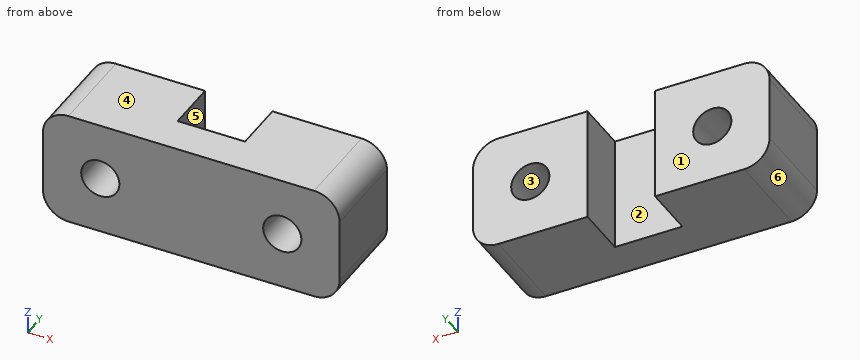
Autodesk Inventor part; units mm, degrees
ref_plane "YZ Plane" through (0, 0, 0) normal (1, 0, 0) x (0, 1, 0)
ref_plane "XZ Plane" through (0, 0, 0) normal (0, 1, 0) x (-1, 0, 0)
ref_plane "XY Plane" through (0, 0, 0) normal (0, 0, 1) x (1, 0, 0)
sketch "Sketch1" plane through (0, 0, 0) normal (0, 0, 1) x (1, 0, 0)
  line L0 (-4.3298, 0.4357) -> (0.9702, 0.4357)
  line L1 (0.9702, 0.4357) -> (0.9702, 4.5357)
  line L2 (-4.3298, 0.4357) -> (-4.3298, 4.5357)
  line L3 (-4.3298, 4.5357) -> (-13.3298, 4.5357)
  line L4 (0.9702, 4.5357) -> (9.9702, 4.5357)
  line L5 (-13.3298, 4.5357) -> (-13.3298, -2.5643)
  line L6 (-13.3298, -2.5643) -> (9.9702, -2.5643)
  line L7 (9.9702, -2.5643) -> (9.9702, 4.5357)
  point P0 (0, 0)
  dimension "d0" = 5.3
  dimension "d1" = 4.1
  dimension "d2" = 9
  dimension "d3" = 9
  dimension "d4" = 3
  dimension "d5" = 4.1
extrude "Extrusion1" add sketch "Sketch1" along normal blind 9
sketch "Sketch2" plane through (-13.3298, 4.5357, 0) normal (0, 1, 0) x (1, 0, 0)
  line L0 (0, 0) -> (9, 0)
  line L1 (0, 0) -> (0, -9)
  line L2 (9, -9) -> (0, -9)
  line L3 (9, 0) -> (9, -9)
  line L4 (14.3, 0) -> (23.3, 0)
  line L5 (14.3, 0) -> (14.3, -9)
  line L6 (23.3, -9) -> (14.3, -9)
  line L7 (23.3, 0) -> (23.3, -9)
  point P0 (13.3298, 0)
  point P1 (4.5, -4.5)
  point P2 (18.8, -4.5)
  dimension "d8" = 9
  dimension "d9" = 9
  dimension "d10" = 4.5
  dimension "d11" = 4.5
  dimension "d12" = 4.5
  dimension "d13" = 4.5
hole "Hole1" at (-8.8298, 4.5357, 4.5) at (5.4702, 4.5357, 4.5) direction (0, -1, 0) diameter 3 end through all
fillet "Fillet1" radius 2 4 edges at (-13.3298, 0.9857, 9) (-13.3298, 0.9857, 0) (9.9702, 0.9857, 0) (9.9702, 0.9857, 9)
equation "\"d5\" = d1"
properties part number "3DP_PLA_Measurement_Rail_Vibration_Motor_Clamp"
Geometry check sheet. Reference: the model listing, model coordinates, mm. Face numbers are marked on the shaded views. A direction names the side the tool comes from. Round coordinates to 2 decimals unless told otherwise and drop trailing zeros. Loops run counter-clockwise (first coordinate to the right, second up) from the corner with the lowest first, then second, coordinate; pieces in that order, holes last. Notation, with made-up numbers: (82.25, -11.5) -> (135.25, -11.5) arc R34 ccw to (135.25, 27.5) -> close; hole circle Ø11 at (82.25, 53). An arc over 180 degrees is marked (long way). Answer as a JSON object with one key per item and string values. Group by question number.
Item 1: Set-up check for the marked faces 1 and 2: record each of +Z, -Z, +X, -X, +Y, -Y from which the full face is reachable in a straight line by a thin tool's end or side.
Item 2: Cross-section at B-B, the plane z = 4.5. Record the cut outline in (x, y).
Item 3: Thickness scan on line 1 along X through (y, z) = (2.5, 4.5); line 2 along X through (y, z) = (0.25, 4.5); line 3 along X through (y, z) = (-1, 4.25). Record the ranges inside material, lowest first.
Item 4: Release check for a two-part mould opening along X. For the marked faces 3, 4, 5 and 6 record: pulls with the +X half, pulls with the -X half, needs draft (parallel to the pull), parting line crosses it, or undercut.
Item 5: Cross-section at D-D, the plane x = -0.25. Record the cut outline in (y, z).
Item 6: Cross-section at C-C, the plane z = 2.75. Record the cut outline in (x, y), plus the area to 3 significant figures.
Item 7: Depth check by flat-ended pin: pin 1 Ø2.5 at (x, z) = (5.47, 4.5) entering from +Y. Enter the tip coordinate at first touch or a pass-through.
Item 8: Cross-section at A-A, the plane y = 2. Record the cut outline in (x, z), plus the area to 3 significant figures.
Determined:
{
 "1": {"face 1": "+Z, -Z, +X, -X, +Y", "face 2": "+Z, -Z, +Y"},
 "2": {"outline": "(-13.33, -2.56) -> (-10.33, -2.56) -> (-10.33, 4.54) -> (-13.33, 4.54) -> close; (-7.33, -2.56) -> (3.97, -2.56) -> (3.97, 4.54) -> (0.97, 4.54) -> (0.97, 0.44) -> (-4.33, 0.44) -> (-4.33, 4.54) -> (-7.33, 4.54) -> close; (6.97, -2.56) -> (9.97, -2.56) -> (9.97, 4.54) -> (6.97, 4.54) -> close"},
 "3": {"line 1": "x = -13.33 to -10.33, -7.33 to -4.33, 0.97 to 3.97, 6.97 to 9.97", "line 2": "x = -13.33 to -10.33, -7.33 to 3.97, 6.97 to 9.97", "line 3": "x = -13.33 to -10.31, -7.35 to 3.99, 6.95 to 9.97"},
 "4": {"face 3": "undercut", "face 4": "needs draft", "face 5": "undercut", "face 6": "pulls with the -X half"},
 "5": {"outline": "(-2.56, 0) -> (0.44, 0) -> (0.44, 9) -> (-2.56, 9) -> close"},
 "6": {"outline": "(-13.33, -2.56) -> (9.97, -2.56) -> (9.97, 4.54) -> (0.97, 4.54) -> (0.97, 0.44) -> (-4.33, 0.44) -> (-4.33, 4.54) -> (-13.33, 4.54) -> close", "area": "144 mm²"},
 "7": {"pin 1": "passes through"},
 "8": {"outline": "(-13.33, 2) arc R2 ccw to (-11.33, 0) -> (-4.33, 0) -> (-4.33, 9) -> (-11.33, 9) arc R2 ccw to (-13.33, 7) -> close; (0.97, 0) -> (7.97, 0) arc R2 ccw to (9.97, 2) -> (9.97, 7) arc R2 ccw to (7.97, 9) -> (0.97, 9) -> close; hole circle Ø3 at (-8.83, 4.5); hole circle Ø3 at (5.47, 4.5)", "area": "144 mm²"}
}
